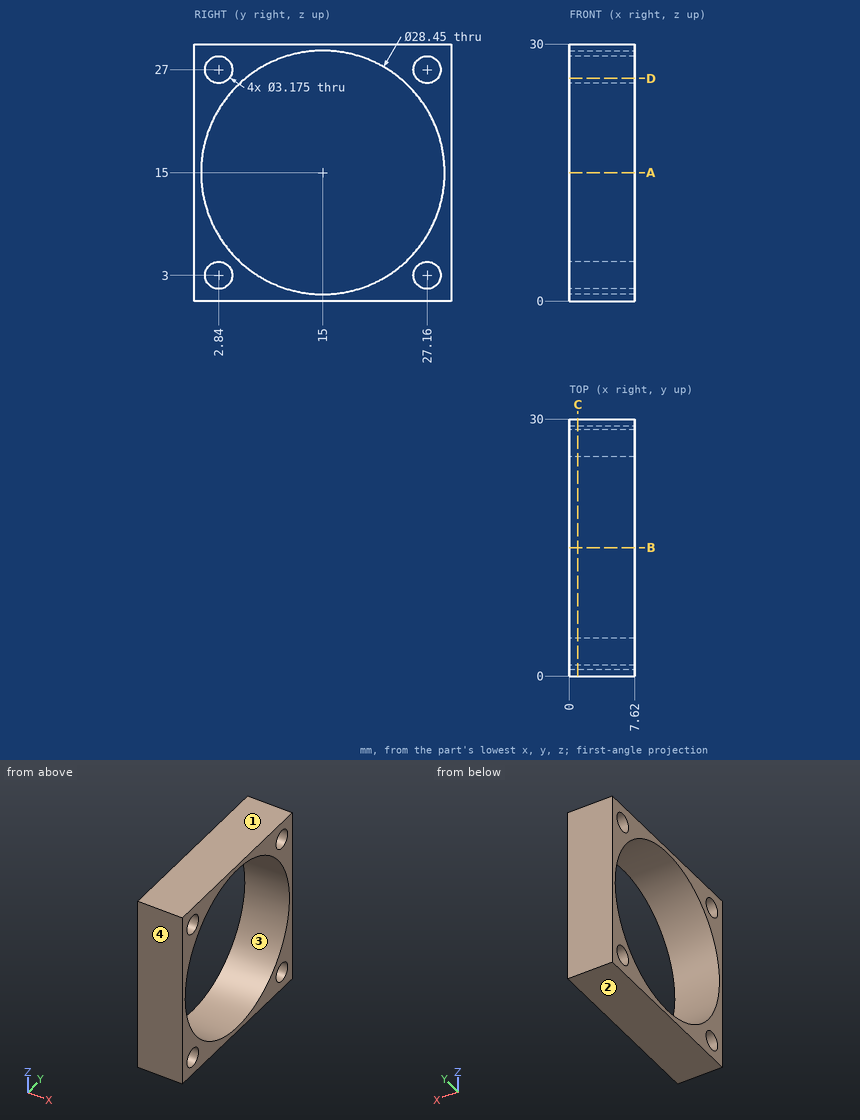
Geometry: see drawing. Coordinates: mm, zero at the bounding-box minimum. Give positions to 0.01 mm unless a question says otherwise; leave off trailing zeros. Loops run counter-clockwise (first coordinate to the right, second up) from the corner with the lowest first, then second, coordinate; pieces in that order, holes last. Notation, with made-up numbers: (-27, 67.5) - (-4, 67.5) arc R33 cw to (-4, 103.5) - close; hole circle Ø2 at (38, -13.75). An arc over 180 degrees is marked (long way). Answer as CSV lines item,"result". Start each with the question number.
1. Section A-A, the plane z = 15. Return loops of the section in (x, y) (3 decimals).
2. Draft query along Z for the marked faces 1, 2, 3 and 4. Return one class per face: released by +Z, released by -Z, zero draft, split by the parting line, or undercut.
3. Section D-D, the plane z = 26. Return loops of the section in (x, y).
4. Ray query, L1, parallel to Z at x = 3, y = 27.16; L2, parallel to Y at x = 5, z = 27; L3, parallel to Z at x = 6, y = 2 (3 decimals). Return the intervals inside material, ascending.
5. Section C-C, the plane x = 1. Give the number of separate pieces and of enclosed holes in the cut face, plus the area to 3 significant figures.
6. Pin query (flat end, axial travel): P1, Ø3, axis at y = 2.84, z = 27, coming from the +X side. Return the tip coordinate at first contact, or that it passes through.
Answers:
1,outline,"(0, 0) - (7.62, 0) - (7.62, 0.775) - (0, 0.775) - close; (0, 29.225) - (7.62, 29.225) - (7.62, 30) - (0, 30) - close"
2,face 1,"released by +Z"
2,face 2,"released by -Z"
2,face 3,"undercut"
2,face 4,"zero draft"
3,outline,"(0, 0) - (7.62, 0) - (7.62, 1.61) - (0, 1.61) - close; (0, 4.07) - (7.62, 4.07) - (7.62, 5.98) - (0, 5.98) - close; (0, 24.02) - (7.62, 24.02) - (7.62, 25.93) - (0, 25.93) - close; (0, 28.39) - (7.62, 28.39) - (7.62, 30) - (0, 30) - close"
4,L1,"z = 0 to 1.41, 4.59 to 7.62, 22.38 to 25.41, 28.59 to 30"
4,L2,"y = 0 to 1.25, 4.43 to 7.36, 22.64 to 25.57, 28.75 to 30"
4,L3,"z = 0 to 1.653, 4.347 to 9.225, 20.775 to 25.653, 28.347 to 30"
5,separate pieces,"1"
5,enclosed holes,"5"
5,area,"233 mm2"
6,P1,"passes through"
